from build123d import *

# Parameters (mm, degrees)
BOSS_EXTRUDE1_DEPTH = 25.4
SKETCH3_R           = 14.2875
SKETCH3_R_2         = 1.7272
CUT_EXTRUDE1_DEPTH  = 54.600169076
SKETCH9_R           = 2.4892
CUT_EXTRUDE2_DEPTH  = 71.995158286


with BuildPart() as part:
    # Sketch2 → Boss-Extrude1 (new, symmetric)
    with BuildSketch(Plane.XY):
        with BuildLine():
            Line((-19.05, -31.75), (19.05, -31.75))
            Line((19.05, -31.75), (19.05, 31.75))
            Line((19.05, 31.75), (17.4625, 31.75))
            ThreePointArc((17.4625, 31.75), (16.339967985, 31.285032015), (15.875, 30.1625))
            Line((15.875, 30.1625), (15.875, -23.7998))
            ThreePointArc((15.875, -23.7998), (14.476376302, -27.176376302), (11.0998, -28.575))
            Line((11.0998, -28.575), (-17.4625, -28.575))
            ThreePointArc((-17.4625, -28.575), (-18.585032015, -29.039967985), (-19.05, -30.1625))
            Line((-19.05, -30.1625), (-19.05, -31.75))
        make_face()
    extrude(amount=BOSS_EXTRUDE1_DEPTH, both=True)

    # Sketch3 → Cut-Extrude1 (cut, through all)
    with BuildSketch(Plane.ZY.offset(-15.875)):
        with Locations(Location((-0.50799991, 3.175, 0), (0, 0, 270))):
            Circle(SKETCH3_R)
        with Locations(Location((12.243963782, 15.926963692, 0), (0, 0, 270))):
            Circle(SKETCH3_R_2)
    extrude(amount=-CUT_EXTRUDE1_DEPTH, mode=Mode.SUBTRACT)

    # Sketch9 → Cut-Extrude2 (cut, through all)
    with BuildSketch(Plane.XZ.offset(31.75)):
        with Locations((0, 15.875)):
            Circle(SKETCH9_R)
        with Locations((0, -15.875)):
            Circle(SKETCH9_R)
    extrude(amount=-CUT_EXTRUDE2_DEPTH, mode=Mode.SUBTRACT)


solid = part.part
The listing builds one solid part. Answer for the finished solid, in the listing's coordinates (mm). A direction names the side the tool comes from. Coordinates: 2 decimals unless noted, no trailing zeros. Write each loop counter-clockwise with the first axis right and the second up, starting at its lowest first coordinate (ties: lowest second). Pieces come first, ordered by that corner, then holes. Notation, with made-up numbers: (82, 68) - (117, 68) arc R23 ccw to (117, 92) - close; hole circle Ø8 at (46.5, 10). An arc over 180 degrees is marked (long way). Return JSON: item names as keys, results as strings.
1. Consider line 1 along Z through (x, y) = (0, -29.25); line 2 along X through (y, z) = (-15, 1) (3 decimals); line 3 along Y through (x, z) = (10.5, -17.5) (3 decimals). Determine where each line is inside the solid, lowest interval first.
Final values:
{"line 1": "-25.4 to -18.36, -13.39 to 13.39, 18.36 to 25.4", "line 2": "15.875 to 19.05", "line 3": "-31.75 to -28.575"}
2. The part is cut by section D-D on x = 8. Determine the outline of the cut face in (y, z) (3 decimals).
Final values:
{"outline": "(-31.75, -25.4) - (-28.575, -25.4) - (-28.575, 25.4) - (-31.75, 25.4) - close"}
3. The part is cut by section C-C on y = 15. Determine the outline of the cut face in (x, z) (3 decimals).
Final values:
{"outline": "(15.875, -25.4) - (19.05, -25.4) - (19.05, -8.527) - (15.875, -8.527) - close; (15.875, 7.511) - (19.05, 7.511) - (19.05, 10.787) - (15.875, 10.787) - close; (15.875, 13.701) - (19.05, 13.701) - (19.05, 25.4) - (15.875, 25.4) - close"}
4. For a pull along X with two mould halves and no side action, classify faces 3 (the face through (-3, -28.575, 0)), 4 (the face through (-0.54, -30.185, -18.305)), 5 (the face through (-18.573, -29.028, 0.356)) as +X half, -X half, draft (parallel to the pull), parting line (faces both ways), or undercut.
Final values:
{"face 3": "draft", "face 4": "undercut", "face 5": "-X half"}
5. Each of these flat-tipped pins is pushed along its axis until it touches: pin 1 Ø2 at (y, z) = (15.93, 12.24) entering from +X; pin 2 Ø10 at (y, z) = (0.5, -15) entering from -X (3 decimals); pin 3 Ø4 at (x, z) = (9, 7) entering from +Y (3 decimals); pin 4 Ø4 at (x, z) = (13.5, -8) entering from +Y. Where does it stop, or does it pass through?
Final values:
{"pin 1": "through", "pin 2": "x = 15.875", "pin 3": "y = -28.575", "pin 4": "y = -25.65"}
6. The part is cut by section A-A on x = 0. Determine the outline of the cut face in (y, z) (3 decimals).
Final values:
{"outline": "(-31.75, -25.4) - (-28.575, -25.4) - (-28.575, -18.364) - (-31.75, -18.364) - close; (-31.75, -13.386) - (-28.575, -13.386) - (-28.575, 13.386) - (-31.75, 13.386) - close; (-31.75, 18.364) - (-28.575, 18.364) - (-28.575, 25.4) - (-31.75, 25.4) - close"}
7. Which of the six approach directions +Z, -Z, +X, -X, +Y, -Y give full straight-line access (tool end or side, diameter ignored) to faces 1 (the face through (17.44, -10.023, -5.98)), 2 (the face through (15.875, -8, -11))?
Final values:
{"face 1": "+X, -X", "face 2": "+Z, -Z, -X, +Y"}
